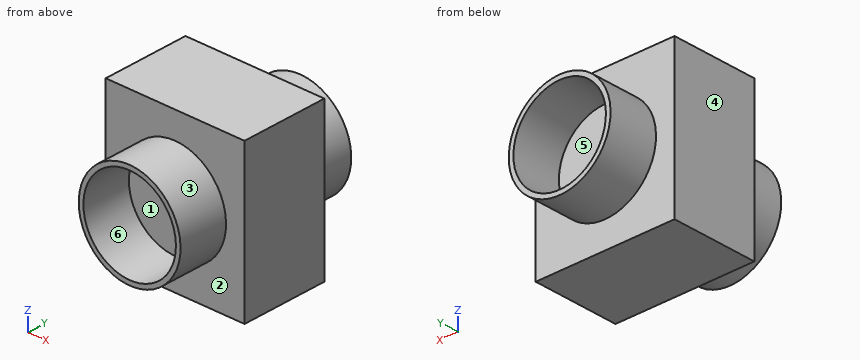
from build123d import *

# Parameters (mm, degrees)
SKETCH1_R           = 11
SKETCH1_R_2         = 10
BOSS_EXTRUDE1_DEPTH = 20
SKETCH2_W           = 33.358065124
SKETCH2_H           = 18.687210396
BOSS_EXTRUDE2_DEPTH = 15


with BuildPart() as part:
    # Sketch1 → Boss-Extrude1 (new, symmetric)
    with BuildSketch(Plane(origin=(0, 0, 0), x_dir=(1, 0, 0), z_dir=(0, 1, 0))):
        with Locations(Location((0, 0, 0), (0, 0, 270))):
            Circle(SKETCH1_R)
        with Locations(Location((0, 0, 0), (0, 0, 270))):
            Circle(SKETCH1_R_2, mode=Mode.SUBTRACT)
    extrude(amount=BOSS_EXTRUDE1_DEPTH, both=True)

    # Sketch2 → Boss-Extrude2 (add, symmetric)
    with BuildSketch(Plane(origin=(0, 0, 0), x_dir=(0, 0, -1), z_dir=(1, 0, 0))):
        Rectangle(SKETCH2_W, SKETCH2_H)
    extrude(amount=BOSS_EXTRUDE2_DEPTH, both=True)


solid = part.part
Model file for the job. Use its own axes, mm. Face numbers are marked on the shaded views. A direction names the side the tool comes from. Give positions to 0.01 mm unless a question says otherwise; leave off trailing zeros. Write each loop counter-clockwise with the first axis right and the second up, starting at its lowest first coordinate (ties: lowest second). Pieces come first, ordered by that corner, then holes. Notation, with made-up numbers: M 25.5,21.25 L 74.5,21.25 A36 cw 74.5,56.25 Z; hole C -22,64.5 d10. An arc over 180 degrees is marked long. One line per item, written item: value. Start each with the question number.
Q1. Saw through at A-A, the plane x = 0. Write the cut outline in (y, z), plus the area to 3 significant figures.
Q2. Two-plate mould, pull along Z, no slides. Class the marked faces 1, 2 and 3: +Z half, -Z half, draft (parallel to the pull), parting line (faces both ways), or undercut.
Q3. Saw through at C-C, the plane z = 0. Write the cut outline in (x, y).
Q4. Drop flat-ended pins along their axis: pin 1 Ø3 at (x, z) = (11.5, 7.5) entering from -Y; pin 2 Ø10 at (x, z) = (1, 2) entering from +Y. Give the stop position or say it passes through.
Q5. Probe probe 1 along X at (y, z) = (15.5, 0); probe 2 along Y at (x, z) = (11, 3); probe 3 along X at (y, z) = (-16, 9). List the from-to ranges inside material, lowest first. Write a range as [from, to].
Q6. Saw through at B-B, the plane y = 17. Write the cut outline in (x, z), plus the area to 3 significant figures.
Q7. 3-axis set-ups, long thin cutter, end or side, ignore diameter. For the marked faces 4, 5 and 6: which of +Z, -Z, +X, -X, +Y, -Y reach the whole face in a straight line?
Output values:
1. outline: M -20,-11 L -9.34,-11 L -9.34,-16.68 L 9.34,-16.68 L 9.34,-11 L 20,-11 L 20,-10 L 9.34,-10 L 9.34,10 L 20,10 L 20,11 L 9.34,11 L 9.34,16.68 L -9.34,16.68 L -9.34,11 L -20,11 L -20,10 L -9.34,10 L -9.34,-10 L -20,-10 Z
1. area: 666 mm²
2. face 1: undercut
2. face 2: draft
2. face 3: parting line
3. outline: M -15,-9.34 L -11,-9.34 L -11,-20 L -10,-20 L -10,-9.34 L 10,-9.34 L 10,-20 L 11,-20 L 11,-9.34 L 15,-9.34 L 15,9.34 L 11,9.34 L 11,20 L 10,20 L 10,9.34 L -10,9.34 L -10,20 L -11,20 L -11,9.34 L -15,9.34 Z
4. pin 1: stops at y = -9.34
4. pin 2: stops at y = 9.34
5. probe 1: x = [-11, -10], [10, 11]
5. probe 2: y = [-9.34, 9.34]
5. probe 3: x = [-6.32, -4.36], [4.36, 6.32]
6. outline: C 0,0 d22; hole C 0,0 d20
6. area: 66.0 mm²
7. face 4: +Z, -Z, -X, +Y, -Y
7. face 5: +Y
7. face 6: -Y
